from build123d import *

# Parameters (mm, degrees)
F1_W     = 42.8306325339
F1_H     = 48.977623228
F2_DEPTH = 1.778
F0_W     = 4.9618608318
F0_H     = 2.4809306487
F3_DEPTH = 8.89


with BuildPart() as f2:
    # F1 (on Top) → F2 (new body)
    with BuildSketch(Plane.XY):
        with Locations((16.6563570965, -3.1726385932)):
            Rectangle(F1_W, F1_H)
    extrude(amount=F2_DEPTH)

    # F0 (on Right) → F3 (join)
    with BuildSketch(Plane.YZ):
        Polygon((4.9618608318, 11.9911627844), (0, 52.7197681367), (0, 11.9911627844), align=None)
        with Locations((2.4809304159, 10.75069746)):
            Rectangle(F0_W, F0_H)
        Polygon((10.337209329, 11.9911627844), (4.9618608318, 11.9911627844), (4.9618608318, 9.5102321357), align=None)
        Polygon((0, 9.5102321357), (0, 11.9911627844), (-8.0630229786, 11.9911627844), align=None)
        Polygon((4.9618608318, 1.6539535718), (4.9618608318, 9.5102321357), (0, 9.5102321357), (0, 1.8606976373), align=None)
    extrude(amount=F3_DEPTH)


solid = f2.part
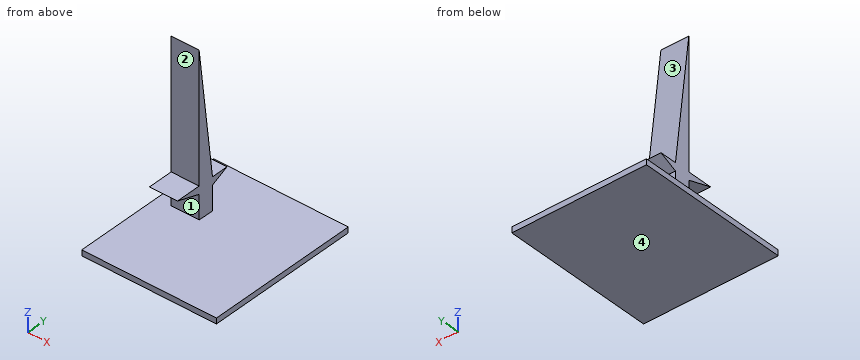
Verification items for the finished model (mm, model axes). Face numbers are marked on the shaded views. Coordinates: 2 decimals unless noted, no trailing zeros. Order: outer loops, then holes, each group sorted by start corner. A loop starts at its lowest first (then second) coordinate and runs counter-clockwise, first axis right, second up.
Item 1: Section check A-A, the plane y = -6.5. Enter the section's corners in (x, z), then the cut area to 3 significant figures.
Filled in:
outline: (-4.76, 0) - (38.07, 0) - (38.07, 1.78) - (-4.76, 1.78) - close; (0, 11.51) - (8.89, 11.51) - (8.89, 11.99) - (0, 11.99) - close
area: 80.4 mm2
Item 2: Depth check by flat-ended pin: pin 1 (2.5 mm diameter, centred on x = 3.5, y = -4.5, fed in from +Z); pin 2 (14.5 mm diameter, centred on y = 5.5, z = 17.5, fed in from -X); pin 3 (2.5 mm diameter, centred on x = 2.5, z = 6.5, fed in from +Y). Enter the tip coordinate at first touch or a pass-through.
Filled in:
pin 1: stops at z = 11.99
pin 2: stops at x = 0
pin 3: stops at y = 4.96
Item 3: Section check B-B, the plane x = 7.5. Enter the section's corners in (y, z).
Filled in:
outline: (-27.66, 0) - (21.32, 0) - (21.32, 1.78) - (4.96, 1.78) - (4.96, 9.51) - (10.34, 11.99) - (4.96, 11.99) - (0, 52.72) - (0, 11.99) - (-8.06, 11.99) - (0, 9.51) - (0, 1.86) - (1.98, 1.78) - (-27.66, 1.78) - close
Item 4: Release check for a two-part mould opening along Z. For the marked faces 1, 2, 3 and 4 record: +Z half, -Z half, draft (parallel to the pull), parting line (faces both ways), or undercut.
Filled in:
face 1: undercut
face 2: draft
face 3: +Z half
face 4: -Z half
Item 5: Section check C-C, the plane y = 6. Enter the section's corners in (x, z).
Filled in:
outline: (-4.76, 0) - (38.07, 0) - (38.07, 1.78) - (-4.76, 1.78) - close; (0, 9.99) - (8.89, 9.99) - (8.89, 11.99) - (0, 11.99) - close
Item 6: Material ranges on L1, parallel to Z at x = 29.5, y = -13.5; L2, parallel to Z at x = 2.5, y = 6; L3, parallel to Y at x = 5, z = 20, recorded low to high.
Filled in:
L1: z = 0 to 1.78
L2: z = 0 to 1.78, 9.99 to 11.99
L3: y = 0 to 3.99
Item 7: Section check D-D, the plane z = 3.5. Enter the section's corners in (x, y), then the cut area to 3 significant figures.
Filled in:
outline: (0, 0) - (8.89, 0) - (8.89, 4.96) - (0, 4.96) - close
area: 44.1 mm2
